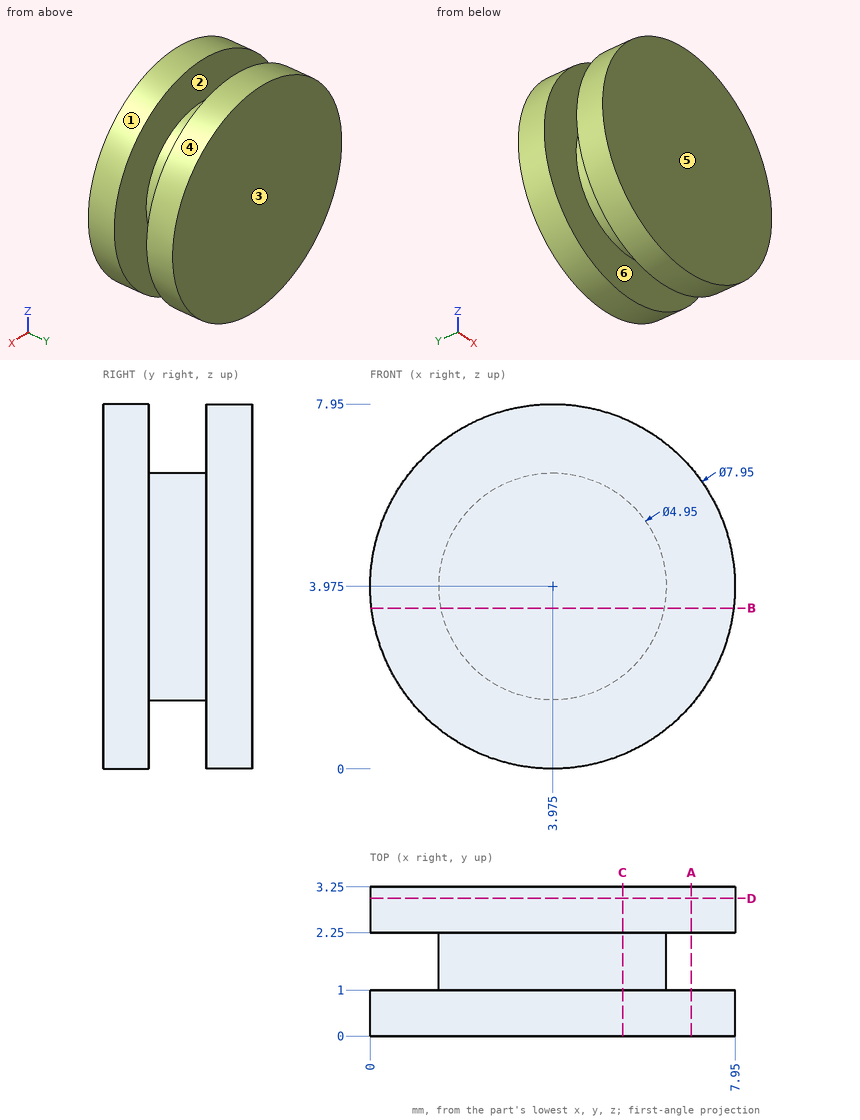
Geometry check sheet. Reference: drawing and pictorial views, mm from the part's lowest x, y, z. A direction names the side the tool comes from. Coordinates: 2 decimals unless noted, no trailing zeros. Order: outer loops, then holes, each group sorted by start corner. A loop starts at its lowest first (then second) coordinate and runs counter-clockwise, first axis right, second up. Notation, with made-up numbers: M 31.5,10.5 L 87.5,10.5 A28 ccw 87.5,40.5 Z; hole C 48,-4.75 d8. An arc over 180 degrees is marked long. Return JSON: item names as keys, results as strings.
1) Thickness scan on L1, parallel to Y at x = 7, z = 5.25; L2, parallel to Z at x = 4, y = 1.15; L3, parallel to Z at x = 5.5, y = 2.55. Record the ranges inside material, lowest first. Write a range as [from, to].
Answer list:
{"L1": "[0, 1], [2.25, 3.25]", "L2": "[1.5, 6.45]", "L3": "[0.3, 7.65]"}
2) Cross-section at C-C, the plane x = 5.5. Record the boundary of the cut face in (y, z).
Answer list:
{"outline": "M 0,0.3 L 1,0.3 L 1,2.03 L 2.25,2.03 L 2.25,0.3 L 3.25,0.3 L 3.25,7.65 L 2.25,7.65 L 2.25,5.92 L 1,5.92 L 1,7.65 L 0,7.65 Z"}
3) Cross-section at B-B, the plane z = 3.5. Record the boundary of the cut face in (x, y).
Answer list:
{"outline": "M 0.03,0 L 7.92,0 L 7.92,1 L 6.4,1 L 6.4,2.25 L 7.92,2.25 L 7.92,3.25 L 0.03,3.25 L 0.03,2.25 L 1.55,2.25 L 1.55,1 L 0.03,1 Z"}
4) Access from +Z, -Z, +X, -X, +Y, -Y to the whole of each face (thin tool, end or side, straight path). Record for the marked faces 1 and 2.
Answer list:
{"face 1": "+Y, -Y", "face 2": "none"}
5) Release check for a two-part mould opening along Y. For the marked faces 3, 4, 5 and 6 record: +Y half, -Y half, draft (parallel to the pull), parting line (faces both ways), or undercut.
Answer list:
{"face 3": "+Y half", "face 4": "draft", "face 5": "-Y half", "face 6": "undercut"}
6) Cross-section at D-D, the plane y = 3. Record the boundary of the cut face in (x, z) (3 decimals).
Answer list:
{"outline": "C 3.975,3.975 d7.95"}
7) Cross-section at A-A, the plane x = 7. Record the boundary of the cut face in (y, z).
Answer list:
{"outline": "M 0,1.4 L 1,1.4 L 1,6.55 L 0,6.55 Z; M 2.25,1.4 L 3.25,1.4 L 3.25,6.55 L 2.25,6.55 Z"}
8) Gauge pin test, flat ends, axial feed: pin 1 (1 mm diameter, centred on y = 2.5, z = 1.5, fed in from -X); pin 2 (1 mm diameter, centred on x = 2, y = 3, fed in from +Z); pin 3 (3 mm diameter, centred on x = 2.5, z = 3, fed in from -Y); pin 4 (1.5 mm diameter, centred on x = 2.5, y = 1.5, fed in from -Z). Record the tip position at first contact, or that the pin passes through.
Answer list:
{"pin 1": "x = 0.53", "pin 2": "z = 7.67", "pin 3": "y = 0", "pin 4": "z = 0.11"}
